Model file for the job. Use its own axes, mm. Coordinates: 2 decimals unless noted, no trailing zeros. Write each loop counter-clockwise with the first axis right and the second up, starting at its lowest first coordinate (ties: lowest second). Pieces come first, ordered by that corner, then holes. Notation, with made-up numbers: (-18.75, -3) - (14.25, -3) arc R20 cw to (14.25, 9) - close; hole circle Ø10 at (32, 59.25). An arc over 180 degrees is marked (long way). Put each result on its own line as item: value. Start each with the question number.
1. Saw through at B-B, the plane x = 28. Write the cut outline in (y, z), plus the area to 3 significant figures.
2. Drop a flat-ended pin along its axis: P1, Ø3, axis at y = 32.5, z = -1.5, coming from the -X side. Give the stop position or say it passes through.
3. Saw through at A-A, the plane z = 2.25. Write the cut outline in (x, y).
4. Drill centre lines: L1, parallel to X at y = 29, z = 1.75; L2, parallel to Z at x = 28, y = -46. Where is each one in solid material? Low to high. Write a range as from..to.
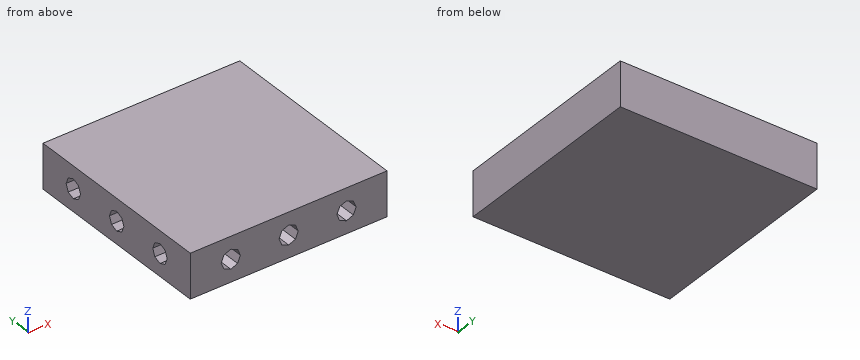
```python
from build123d import *

# Parameters (mm, degrees)
F0_W     = 102
F0_H     = 23
F1_DEPTH = 51
F3_DEPTH = 10
F5_DEPTH = 10


with BuildPart() as f1:
    # F0 (on Right) → F1 (new body, symmetric)
    with BuildSketch(Plane.YZ):
        Rectangle(F0_W, F0_H)
    extrude(amount=F1_DEPTH, both=True)

    # F2 (on face) → F3 (cut)
    with BuildSketch(Plane.XZ.offset(51)):
        Polygon((3.535534, -3.535534), (5, 0), (3.535534, 3.535534), (0, 5), (-3.535534, 3.535534), (-5, 0), (-3.535534, -3.535534), (0, -5), align=None)
        Polygon((33.535534, 3.535534), (30, 5), (26.464466, 3.535534), (25, 0), (26.464466, -3.535534), (30, -5), (33.535534, -3.535534), (35, 0), align=None)
        Polygon((-26.464466, 3.535534), (-30, 5), (-33.535534, 3.535534), (-35, 0), (-33.535534, -3.535534), (-30, -5), (-26.464466, -3.535534), (-25, 0), align=None)
    extrude(amount=-F3_DEPTH, mode=Mode.SUBTRACT)

    # F4 (on face) → F5 (cut)
    with BuildSketch(Plane(origin=(-51, 0, 0), x_dir=(0, -1, 0), z_dir=(-1, 0, 0))):
        Polygon((3.535534, -3.535534), (5, 0), (3.535534, 3.535534), (0, 5), (-3.535534, 3.535534), (-5, 0), (-3.535534, -3.535534), (0, -5), align=None)
        Polygon((30, 5), (26.464466, 3.535534), (25, 0), (26.464466, -3.535534), (30, -5), (33.535534, -3.535534), (35, 0), (33.535534, 3.535534), align=None)
        Polygon((-25, 0), (-26.464466, 3.535534), (-30, 5), (-33.535534, 3.535534), (-35, 0), (-33.535534, -3.535534), (-30, -5), (-26.464466, -3.535534), align=None)
    extrude(amount=-F5_DEPTH, mode=Mode.SUBTRACT)


with BuildPart() as f6_1:
    # F6: copy of F1
    add(f1.part)


solid = f1.part
```
Final values:
1. outline: (-51, -11.5) - (51, -11.5) - (51, 11.5) - (-51, 11.5) - (-51, 4.17) - (-41, 4.17) - (-41, -4.17) - (-51, -4.17) - close
1. area: 2,260 mm²
2. P1: stops at x = -41
3. outline: (-51, -51) - (-34.07, -51) - (-34.07, -41) - (-25.93, -41) - (-25.93, -51) - (-4.07, -51) - (-4.07, -41) - (4.07, -41) - (4.07, -51) - (25.93, -51) - (25.93, -41) - (34.07, -41) - (34.07, -51) - (51, -51) - (51, 51) - (-51, 51) - (-51, 34.07) - (-41, 34.07) - (-41, 25.93) - (-51, 25.93) - (-51, 4.07) - (-41, 4.07) - (-41, -4.07) - (-51, -4.07) - (-51, -25.93) - (-41, -25.93) - (-41, -34.07) - (-51, -34.07) - close
4. L1: x = -41..51
4. L2: z = -11.5..-4.17, 4.17..11.5
